Geometry: final body of the model. Coordinates: model frame, mm. Give positions to 0.01 mm unless a question says otherwise; leave off trailing zeros. Loops run counter-clockwise (first coordinate to the right, second up) from the corner with the lowest first, then second, coordinate; pieces in that order, holes last.
```python
from build123d import *

# Parameters (mm, degrees)
CROQUIS1_R              = 2.1
SALIENTE_EXTRUIR1_DEPTH = 6.35
CROQUIS2_R              = 2.75
CROQUIS2_R_2            = 17.4625
CROQUIS2_R_3            = 2.5
CORTAR_EXTRUIR1_DEPTH   = 12.7


with BuildPart() as part:
    # Croquis1 → Saliente-Extruir1 (new body)
    with BuildSketch(Plane.XY):
        Polygon((0, 0), (0, 82.389877484), (-120.421799317, 310.14248627), (-219.400809699, 310.14248627), (-219.400809699, 200), (-103.153458954, -19.85751373), (0, -19.85751373), align=None)
        with Locations((-40.1, 81.05)):
            Circle(CROQUIS1_R, mode=Mode.SUBTRACT)
        with Locations((-10, 81.05)):
            Circle(CROQUIS1_R, mode=Mode.SUBTRACT)
        with Locations((-10, 48.95)):
            Circle(CROQUIS1_R, mode=Mode.SUBTRACT)
        with Locations((-40.1, 48.95)):
            Circle(CROQUIS1_R, mode=Mode.SUBTRACT)
        with Locations((-130, 81.05)):
            Circle(CROQUIS1_R, mode=Mode.SUBTRACT)
        with Locations((-99.9, 81.05)):
            Circle(CROQUIS1_R, mode=Mode.SUBTRACT)
        with Locations((-99.9, 48.95)):
            Circle(CROQUIS1_R, mode=Mode.SUBTRACT)
        with Locations((-130, 48.95)):
            Circle(CROQUIS1_R, mode=Mode.SUBTRACT)
        with Locations((-70, 24.15)):
            Circle(CROQUIS1_R, mode=Mode.SUBTRACT)
        with Locations((-70, -7.95)):
            Circle(CROQUIS1_R, mode=Mode.SUBTRACT)
    extrude(amount=SALIENTE_EXTRUIR1_DEPTH)

    # Croquis2 → Cortar-Extruir1 (cut)
    with BuildSketch(Plane.XY.offset(6.35)):
        with Locations((-212.545809699, 258.28748627)):
            Circle(CROQUIS2_R)
        with Locations((-212.545809699, 211.99748627)):
            Circle(CROQUIS2_R)
        with Locations((-166.255809699, 211.99748627)):
            Circle(CROQUIS2_R)
        with Locations((-166.255809699, 258.28748627)):
            Circle(CROQUIS2_R)
        with Locations((-189.400809699, 235.14248627)):
            Circle(CROQUIS2_R_2)
        with Locations((-129.400809699, 235.14248627)):
            Circle(CROQUIS2_R_3)
        with Locations((-129.400809699, 301.14248627)):
            Circle(CROQUIS2_R_3)
    extrude(amount=-CORTAR_EXTRUIR1_DEPTH, mode=Mode.SUBTRACT)


solid = part.part
```
Q1. Section query C-C, the plane x = -88.5. Return loops of the section in (y, z).
Q2. Pin query (flat end, axial travel): pin 1 Ø4 at (x, y) = (-99.9, 48.95) entering from +Z; pin 2 Ø1.5 at (x, z) = (-131, 3) entering from -Y. Return the tip coordinate at first contact, or that it passes through.
Q3. Section query B-B, the plane y = 265.5. Return loops of the section in (x, z), and give its area (3 significant figures).
Q4. Mould query, pull axis Y, two halves, no side actions, for faces 1 (the face through (-52, -19.858, 3)), 2 (the face through (-59.368, 194.672, 3.131)), 3 (the face through (-219.401, 256, 3)), 4 (the face through (-181.34, 219.65, 3.22)). Classes: +Y half, -Y half, draft (parallel to the pull), parting line (faces both ways), or undercut.
Q5. Material intervals for probe 1 along Y at (x, z) = (-99.9, 5); probe 2 along X at (y, z) = (257.5, 4.75); probe 3 along Y at (x, z) = (-40.1, 4.25), sorted ascending.
Q6. Section query A-A, the plane z = 4.25. State how many separate pieces and enclosed holes the cut face has, and give its area (3 significant figures).
Resolved:
1. outline: (-19.86, 0) - (249.77, 0) - (249.77, 6.35) - (-19.86, 6.35) - close
2. pin 1: passes through
2. pin 2: stops at y = 31.39
3. outline: (-219.4, 0) - (-96.82, 0) - (-96.82, 6.35) - (-219.4, 6.35) - close
3. area: 778 mm2
4. face 1: -Y half
4. face 2: +Y half
4. face 3: draft
4. face 4: undercut
5. probe 1: y = -19.86 to 46.85, 51.05 to 78.95, 83.15 to 271.33
5. probe 2: x = -219.4 to -215.18, -209.91 to -168.89, -163.62 to -92.59
5. probe 3: y = -19.86 to 46.85, 51.05 to 78.95, 83.15 to 158.23
6. separate pieces: 1
6. enclosed holes: 17
6. area: 44,700 mm2
